from build123d import *

# Parameters (mm, degrees)
ESQUISSE1_W        = 88
ESQUISSE1_H        = 20
ESQUISSE1_R        = 1.75
BOSS_EXTRU_1_DEPTH = 3
ESQUISSE2_W        = 60
ESQUISSE2_H        = 3
BOSS_EXTRU_2_DEPTH = 5
CONG_1_R           = 3


with BuildPart() as part:
    # Esquisse1 → Boss.-Extru.1 (new body)
    with BuildSketch(Plane.XY):
        with Locations((44, 10)):
            Rectangle(ESQUISSE1_W, ESQUISSE1_H)
        with Locations((2.5, 10)):
            Circle(ESQUISSE1_R, mode=Mode.SUBTRACT)
        with Locations((85.5, 10)):
            Circle(ESQUISSE1_R, mode=Mode.SUBTRACT)
    extrude(amount=BOSS_EXTRU_1_DEPTH)

    # Esquisse2 → Boss.-Extru.2 (add)
    with BuildSketch(Plane.XY.offset(3)):
        with Locations((44, 10)):
            Rectangle(ESQUISSE2_W, ESQUISSE2_H)
    extrude(amount=BOSS_EXTRU_2_DEPTH)

    # Congé1
    cong_1_edges = [part.edges().sort_by_distance(p)[0] for p in [
        (0, 20, 1.5),
        (88, 20, 1.5),
        (88, 0, 1.5),
        (0, 0, 1.5),
    ]]
    fillet(cong_1_edges, radius=CONG_1_R)


solid = part.part
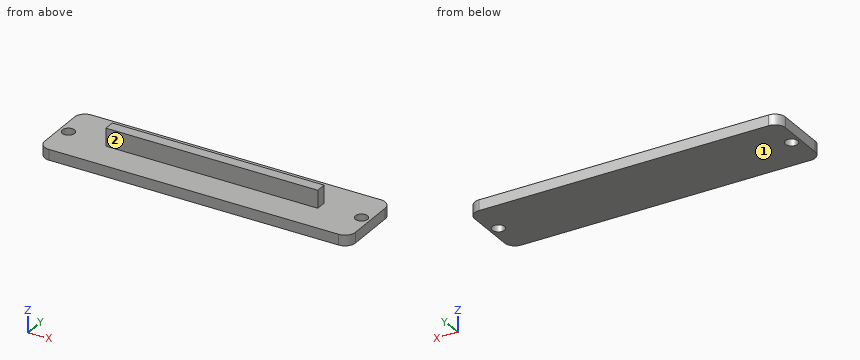
Model file for the job. Use its own axes, mm. Face numbers are marked on the shaded views. A direction names the side the tool comes from. Give positions to 0.01 mm unless a question says otherwise; leave off trailing zeros. Loops run counter-clockwise (first coordinate to the right, second up) from the corner with the lowest first, then second, coordinate; pieces in that order, holes last. Notation, with made-up numbers: (-31.75, 50) - (4.25, 50) arc R31 ccw to (4.25, 81) - close; hole circle Ø9 at (62.5, 8). An arc over 180 degrees is marked (long way). Use one line per item in the form item = value.
(1) Drill centre lines: L1, parallel to Z at x = 19.5, y = 2.5; L2, parallel to Y at x = 34, z = 5.25; L3, parallel to Y at x = 2.5, z = 0.6. Where is each one in solid material? Low to high.
Determined:
L1 = 0 to 3
L2 = 8.5 to 11.5
L3 = 0.04 to 8.25, 11.75 to 19.96
(2) 3-axis set-ups, long thin cutter, end or side, ignore diameter. For the marked faces 1 and 2: which of +Z, -Z, +X, -X, +Y, -Y reach the whole face in a straight line?
Determined:
face_1 = -Z, +X, -X, +Y, -Y
face_2 = +Z, +X, -X, -Y
(3) Cut at A-A (y = 10). Give the cut face in (x, z).
Determined:
outline = (0, 0) - (0.75, 0) - (0.75, 3) - (0, 3) - close; (4.25, 0) - (83.75, 0) - (83.75, 3) - (74, 3) - (74, 8) - (14, 8) - (14, 3) - (4.25, 3) - close; (87.25, 0) - (88, 0) - (88, 3) - (87.25, 3) - close
(4) Cut at C-C (z = 4.5). Give the cut face in (x, y), then the cut area to 3 significant figures.
Determined:
outline = (14, 8.5) - (74, 8.5) - (74, 11.5) - (14, 11.5) - close
area = 180 mm^2
(5) Cut at D-D (y = 4). Give the cut face in (x, z).
Determined:
outline = (0, 0) - (88, 0) - (88, 3) - (0, 3) - close
(6) Drop flat-ended pins along their axis: P1, Ø4, axis at x = 85.5, y = 10, coming from the -Z side; P2, Ø0.9, axis at y = 10, z = 5, coming from the -X side; P3, Ø3.5, axis at y = 9.5, z = 5.5, coming from the +X side; P4, Ø5, axis at x = 36.5, y = 2.5, coming from the +Z side. Give the stop position or say it passes through.
Determined:
P1 = 0
P2 = 14
P3 = 74
P4 = 3
(7) Cut at B-B (x = 20). Give the cut face in (y, z).
Determined:
outline = (0, 0) - (20, 0) - (20, 3) - (11.5, 3) - (11.5, 8) - (8.5, 8) - (8.5, 3) - (0, 3) - close
